```python
from build123d import *

# Parameters (mm, degrees)
SKETCH_1_R          = 5.5
EXTRUDE_1_DEPTH     = 15
SKETCH_2_R          = 35
CUT_EXTRUDE_1_DEPTH = 10
SKETCH_3_R          = 10
CUT_EXTRUDE_2_DEPTH = 18.58835
SKETCH_5_R          = 9
EXTRUDE_2_DEPTH     = 12.5
EXTRUDE_3_DEPTH     = 6


with BuildPart() as part:
    # Эскиз1 → Бобышка-Вытянуть1 (new body)
    with BuildSketch(Plane(origin=(0, 0, 0), x_dir=(1, 0, 0), z_dir=(0, 1, 0))):
        with BuildLine():
            Line((42.5, -52.5), (-42.5, -52.5))
            ThreePointArc((-42.5, -52.5), (-49.571067812, -49.571067812), (-52.5, -42.5))
            Line((-52.5, -42.5), (-52.5, 42.5))
            ThreePointArc((-52.5, 42.5), (-49.571067812, 49.571067812), (-42.5, 52.5))
            Line((-42.5, 52.5), (42.5, 52.5))
            ThreePointArc((42.5, 52.5), (49.571067812, 49.571067812), (52.5, 42.5))
            Line((52.5, 42.5), (52.5, -42.5))
            ThreePointArc((52.5, -42.5), (49.571067812, -49.571067812), (42.5, -52.5))
        make_face()
        with Locations(Location((-40, -40, 0), (0, 0, 270))):
            Circle(SKETCH_1_R, mode=Mode.SUBTRACT)
        with Locations(Location((-40, 40, 0), (0, 0, 270))):
            Circle(SKETCH_1_R, mode=Mode.SUBTRACT)
        with Locations(Location((40, 40, 0), (0, 0, 270))):
            Circle(SKETCH_1_R, mode=Mode.SUBTRACT)
        with Locations(Location((40, -40, 0), (0, 0, 270))):
            Circle(SKETCH_1_R, mode=Mode.SUBTRACT)
    extrude(amount=EXTRUDE_1_DEPTH)

    # Эскиз2 → Вырез-Вытянуть1 (cut)
    with BuildSketch(Plane.XZ):
        with Locations(Location((0, 0, 0), (0, 0, 270))):
            Circle(SKETCH_2_R)
    extrude(amount=-CUT_EXTRUDE_1_DEPTH, mode=Mode.SUBTRACT)

    # Эскиз3 → Вырез-Вытянуть2 (cut)
    with BuildSketch(Plane.XY.offset(-52.5)):
        with Locations((0, -5)):
            Circle(SKETCH_3_R)
    extrude(amount=CUT_EXTRUDE_2_DEPTH, mode=Mode.SUBTRACT)

    # Эскиз5 → Бобышка-Вытянуть2 (add, symmetric)
    with BuildSketch(Plane(origin=(0, 0, 0), x_dir=(0, 0, -1), z_dir=(1, 0, 0))):
        with BuildLine():
            Line((15, 45), (15, 15))
            Line((15, 15), (-15, 15))
            Line((-15, 15), (-15, 45))
            ThreePointArc((-15, 45), (0, 60), (15, 45))
        make_face()
        with Locations((0, 45)):
            Circle(SKETCH_5_R, mode=Mode.SUBTRACT)
    extrude(amount=EXTRUDE_2_DEPTH, both=True)

    # Эскиз7 → Бобышка-Вытянуть3 (add, symmetric)
    with BuildSketch(Plane(origin=(0, 0, 0), x_dir=(0, 0, -1), z_dir=(1, 0, 0))):
        Polygon((52.5, 15), (10.44023047, 55.770403323), (10.44023047, 15), align=None)
        Polygon((-52.5, 15), (-10.44023047, 55.770403323), (-10.44023047, 15), align=None)
    extrude(amount=EXTRUDE_3_DEPTH, both=True)


solid = part.part
```
Input: part model. Units: mm. Frame: model coordinates. A direction names the side the tool comes from. Round coordinates to 2 decimals unless told otherwise and drop trailing zeros. Write each loop counter-clockwise with the first axis right and the second up, starting at its lowest first coordinate (ties: lowest second). Pieces come first, ordered by that corner, then holes. Notation, with made-up numbers: (17.25, 23.5) -> (31.25, 23.5) arc R28 ccw to (31.25, 43.5) -> close; hole circle Ø6 at (73.25, 11). An arc over 180 degrees is marked (long way). Answer as CSV lines item,"result".
1. Ray query, L1, parallel to X at y = 9, z = 40; L2, parallel to Y at x = 0.75, z = 0; L3, parallel to X at y = 40, z = -20. Return the intervals inside material, ascending. Write a range as [from, to].
Geometry says:
L1,"x = [-52.5, -45.5], [-34.5, 34.5], [45.5, 52.5]"
L2,"y = [10, 36], [54, 60]"
L3,"x = [-6, 6]"
2. Section D-D (x = 0). Return the cut outline in (y, z).
Geometry says:
outline,"(0, 35) -> (10, 35) -> (10, -35) -> (5, -35) -> (5, -52.5) -> (15, -52.5) -> (55.77, -10.44) arc R15 ccw to (55.77, 10.44) -> (15, 52.5) -> (0, 52.5) -> close; hole circle Ø18 at (45, 0)"
3. Section C-C (y = 12.5). Return the cut outline in (x, z), plus the area to 3 significant figures.
Geometry says:
outline,"(-52.5, -42.5) arc R10 ccw to (-42.5, -52.5) -> (42.5, -52.5) arc R10 ccw to (52.5, -42.5) -> (52.5, 42.5) arc R10 ccw to (42.5, 52.5) -> (-42.5, 52.5) arc R10 ccw to (-52.5, 42.5) -> close; hole circle Ø11 at (-40, -40); hole circle Ø11 at (-40, 40); hole circle Ø11 at (40, -40); hole circle Ø11 at (40, 40)"
area,"10,600 mm^2"
4. Mould query, pull axis Z, two halves, no side actions, for faces 1 (the flat face through (0.084, 35.1, 31.765)), 2 (the cylindrical face through (40.242, 7.395, 34.505)), 3 (the flat face through (12.5, 33, 0)). Classes: +Z half, -Z half, draft (parallel to the pull), parting line (faces both ways), or undercut.
Geometry says:
face 1,"+Z half"
face 2,"undercut"
face 3,"draft"
5. Reachability of faces 4 (the flat face through (9, 30, -15)), 5 (the flat face through (6, 26, 27)), 6 (the flat face through (-6, 26, -27)), 7 (the flat face through (0, 10, 0)), 8 (the flat face through (-9, 30, 15)) from +Z, -Z, +X, -X, +Y, -Y: full face, straight path, thin tool, end or side. Return the list, or none.
Geometry says:
face 4,"-Z, +X, +Y"
face 5,"+Z, +X, +Y"
face 6,"-Z, -X, +Y"
face 7,"-Y"
face 8,"+Z, -X, +Y"
6. Contact query for flat-ended pins moving along their axis: P1, Ø14.5, axis at x = -40, z = -40, coming from the +Y side; P2, Ø12, axis at y = 44.5, z = -35.5, coming from the +X side; P3, Ø14.5, axis at x = 40, z = 40, coming from the -Y side; P4, Ø1.5, axis at x = -7.5, y = 29, coming from the +Z side. Output: stop coordinate, or through.
Geometry says:
P1,"stops at y = 15"
P2,"passes through"
P3,"stops at y = 0"
P4,"stops at z = 15"
7. Section A-A (x = -40). Return the cut outline in (y, z), plus the area to 4 significant figures.
Geometry says:
outline,"(0, -52.5) -> (15, -52.5) -> (15, -45.5) -> (0, -45.5) -> close; (0, -34.5) -> (15, -34.5) -> (15, 34.5) -> (0, 34.5) -> close; (0, 45.5) -> (15, 45.5) -> (15, 52.5) -> (0, 52.5) -> close"
area,"1,245 mm^2"
8. Section B-B (z = 0). Return the cut outline in (x, y).
Geometry says:
outline,"(-52.5, 0) -> (-35, 0) -> (-35, 10) -> (35, 10) -> (35, 0) -> (52.5, 0) -> (52.5, 15) -> (12.5, 15) -> (12.5, 36) -> (-12.5, 36) -> (-12.5, 15) -> (-52.5, 15) -> close; (-12.5, 54) -> (12.5, 54) -> (12.5, 60) -> (-12.5, 60) -> close"
